Build history of the part. All positions in model axes, mm. A direction names the side the tool comes from. Round coordinates to 2 decimals unless told otherwise and drop trailing zeros. Loops run counter-clockwise (first coordinate to the right, second up) from the corner with the lowest first, then second, coordinate; pieces in that order, holes last. Notation, with made-up numbers: M 55.5,-8 L 67.5,-8 A22 cw 67.5,6 Z; hole C 14,17 d3. An arc over 180 degrees is marked long. One line per item, written item: value.
```python
from build123d import *

# Parameters (mm, degrees)
F1_DEPTH = 25
F2_R     = 12.5
F3_DEPTH = 2
F4_SIZE  = 5


with BuildPart() as f1:
    # F0 (on Top) → F1 (new body)
    with BuildSketch(Plane.XY):
        with BuildLine():
            Line((17.320508, 30), (-17.320508, 30))
            ThreePointArc((-17.320508, 30), (-34.641016, 20), (-34.641016, 0))
            Line((-34.641016, 0), (-17.320508, -30))
            ThreePointArc((-17.320508, -30), (0, -40), (17.320508, -30))
            Line((17.320508, -30), (34.641016, 0))
            ThreePointArc((34.641016, 0), (34.641016, 20), (17.320508, 30))
        make_face()
    extrude(amount=F1_DEPTH)

    # F2 (on face) → F3 (cut)
    with BuildSketch(Plane.XY.offset(25)):
        with Locations((-17.320508, 10)):
            Circle(F2_R)
        with Locations((0, -20)):
            Circle(F2_R)
        with Locations((17.320508, 10)):
            Circle(F2_R)
    extrude(amount=-F3_DEPTH, mode=Mode.SUBTRACT)

    # F4
    f4_edges = [f1.edges().sort_by_distance(p)[0] for p in [
        (25.980762, -15, 25),
    ]]
    chamfer(f4_edges, length=F4_SIZE)


solid = f1.part
```
Item 1: Which spindle directions (+Z, -Z, +X, -X, +Y, -Y) get a long thin tool onto all of the face, cutting with end or side? Do faces 1 (the face through (-30.95, 18.13, 24.13)), 2 (the face through (-27.24, 2.394, 24.014)). Say none if no direction does.
Check values:
face 1: +Z, -X
face 2: +Z
Item 2: Wall check: line 1 along Z through (x, y) = (-18.5, 21); line 2 along Y through (x, z) = (0.5, 6.25); line 3 along Y through (x, z) = (0, 23.9). Give the ranges that are in metal, low to high.
Check values:
line 1: z = 0 to 23
line 2: y = -39.99 to 30
line 3: y = -36.1 to -32.5, -7.5 to 26.1
Item 3: Drop flat-ended pins along their axis: P1, Ø1.5, axis at x = -6.5, y = -17.5, coming from the +Z side; P2, Ø8, axis at x = -26, z = 12, coming from the -Y side; P3, Ø12, axis at y = -5, z = 15, coming from the -X side. Give the stop position or say it passes through.
Check values:
P1: stops at z = 23
P2: stops at y = -21.89
P3: stops at x = -35.18
Item 4: Slice it at C-C, the plane z = 10.5. Give the cut face in (x, y), and give its area (3 significant figures).
Check values:
outline: M -34.64,0 L -17.32,-30 A20 ccw 17.32,-30 L 34.64,0 A20 ccw 17.32,30 L -17.32,30 A20 ccw Z
area: 3,850 mm2
Item 5: Slice it at D-D, the plane y = -20. Give the cut face in (x, z).
Check values:
outline: M -23.09,0 L 23.09,0 L 23.09,20 L 17.32,25 L 12.5,25 L 12.5,23 L -12.5,23 L -12.5,25 L -17.32,25 L -23.09,20 Z
Item 6: Pull direction X, two halves, no side cores. Call faces 3 (the face through (31.18, 17.73, 24.13)), 4 (the face through (0, 2, 25)), 5 (the face through (-17, 10, 23)): pulls with the +X half, pulls with the -X half, needs draft (parallel to the pull), parting line crosses it, or undercut.
Check values:
face 3: pulls with the +X half
face 4: needs draft
face 5: undercut
Item 7: Slice it at A-A, the plane y = 10. Give the cut face in (x, z).
Check values:
outline: M -37.32,0 L 37.32,0 L 37.32,20 L 32.32,25 L 29.82,25 L 29.82,23 L 4.82,23 L 4.82,25 L -4.82,25 L -4.82,23 L -29.82,23 L -29.82,25 L -32.32,25 L -37.32,20 Z
Item 8: Slice it at B-B, the plane x = 0. Give the cut face in (y, z), and give its area (4 significant figures).
Check values:
outline: M -40,0 L 30,0 L 30,20 L 25,25 L -7.5,25 L -7.5,23 L -32.5,23 L -32.5,25 L -35,25 L -40,20 Z
area: 1,675 mm2
